Autodesk Inventor part; units mm, degrees
ref_plane "YZ Plane" through (0, 0, 0) normal (1, 0, 0) x (0, 1, 0)
ref_plane "XZ Plane" through (0, 0, 0) normal (0, 1, 0) x (-1, 0, 0)
ref_plane "XY Plane" through (0, 0, 0) normal (0, 0, 1) x (1, 0, 0)
sketch "Sketch1" plane through (0, 0, 0) normal (0, 0, 1) x (1, 0, 0)
  line L0 (0, 0) -> (25, 0)
  line L1 (25, 0) -> (25, 3)
  line L2 (0, 3) -> (25, 3)
  line L3 (0, 0) -> (0, 3)
  line L4 (25, 0) -> (50, 0)
  line L5 (50, 0) -> (50, 3)
  line L6 (25, 3) -> (50, 3)
  line L7 (25, 0) -> (25, 3)
  line L8 (50, 0) -> (75, 0)
  line L9 (75, 0) -> (75, 3)
  line L10 (50, 3) -> (75, 3)
  line L11 (50, 0) -> (50, 3)
  line L12 (0, 0) -> (0, 75)
  line L13 (0, 75) -> (75, 75)
  line L14 (75, 75) -> (75, 0)
  line L15 (75, 0) -> (50, 0)
  line L16 (50, 3) -> (50, 0)
  line L17 (50, 3) -> (25, 3)
  line L18 (25, 3) -> (25, 0)
  line L19 (25, 0) -> (0, 0)
  line L20 (0, 0) -> (0, 25)
  line L21 (0, 25) -> (3, 25)
  line L22 (3, 25) -> (3, 50)
  line L23 (3, 50) -> (0, 50)
  line L24 (25, 75) -> (25, 72)
  line L25 (25, 72) -> (50, 72)
  line L26 (50, 75) -> (50, 72)
  line L27 (75, 50) -> (72, 50)
  line L28 (72, 50) -> (72, 25)
  line L29 (72, 25) -> (75, 25)
  dimension "d0" = 75
  dimension "d1" = 75
  dimension "d2" = 25
  dimension "d3" = 3
  dimension "d4" = 25
  dimension "d5" = 3
  dimension "d6" = 3
extrude "Extrusion1" add sketch "Sketch1" along normal blind 3 contours L3 L2 L1 L0 | L12 L21 L22 L23 L13 L24 L25 L26 L14 L27 L28 L29 L10 L6 L2 | L5 L10 L9 L8
sketch "Sketch2" plane through (0, 0, 0) normal (0, 0, -1) x (-1, 0, 0)
  circle A0 centre (-72, 55.2929) radius 1.5
  circle A1 centre (-20, 68.5) radius 1.5
  circle A2 centre (-23, 21.5) radius 1.5
  circle A3 centre (-72, 23.7071) radius 1.5
  point P0 (0, 0)
extrude "Extrusion2" cut sketch "Sketch2" against normal blind 25.4
sketch "Sketch3" plane through (0, 0, 0) normal (0, 0, -1) x (-1, 0, 0)
  line L0 (-50, 72) -> (-39, 72)
  line L1 (-25, 72) -> (-25, 75)
  line L2 (-25, 75) -> (0, 75)
  line L3 (0, 62.5) -> (0, 50)
  line L4 (0, 50) -> (-3, 50)
  line L5 (-3, 50) -> (-3, 39)
  line L6 (-3, 25) -> (0, 25)
  line L7 (0, 25) -> (0, 0)
  line L8 (0, 0) -> (-25, 0)
  line L9 (-25, 0) -> (-25, 3)
  line L10 (-25, 3) -> (-36, 3)
  line L11 (-50, 3) -> (-50, 0)
  line L12 (-50, 0) -> (-75, 0)
  line L13 (-75, 0) -> (-75, 25)
  line L14 (-75, 25) -> (-72, 25)
  line L15 (-72, 25) -> (-72, 36)
  line L16 (-72, 50) -> (-75, 50)
  line L17 (-75, 62.5) -> (-75, 75)
  line L18 (-75, 75) -> (-50, 75)
  line L19 (-50, 75) -> (-50, 72)
  circle A0 centre (-19, 19.65) radius 1.5
  circle A1 centre (-19, 56.95) radius 1.5
  circle A2 centre (-56.3, 56.95) radius 1.5
  circle A3 centre (-56.3, 19.65) radius 1.5
  line L20 (-39, 72) -> (-36, 72)
  line L21 (-3, 39) -> (-3, 36)
  line L22 (-3, 50) -> (-3, 25)
  line L23 (-39, 3) -> (-36, 3)
  line L24 (-25, 3) -> (-50, 3)
  line L25 (-72, 36) -> (-72, 39)
  line L26 (-72, 25.2071) -> (-72, 50)
  line L27 (-72, 39) -> (-72, 50)
  line L28 (-36, 72) -> (-25, 72)
  line L29 (-3, 36) -> (-3, 25)
  line L30 (-39, 3) -> (-50, 3)
  line L31 (-72, 36) -> (-65.65, 36)
  line L32 (-65.65, 36) -> (-65.65, 34)
  line L33 (-65.65, 34) -> (-63.15, 34)
  line L34 (-63.15, 34) -> (-63.15, 36)
  line L35 (-63.15, 36) -> (-59.3, 36)
  line L36 (-59.3, 36) -> (-59.3, 39)
  line L37 (-59.3, 39) -> (-63.15, 39)
  line L38 (-63.15, 39) -> (-63.15, 41)
  line L39 (-63.15, 41) -> (-65.65, 41)
  line L40 (-65.65, 41) -> (-65.65, 39)
  line L41 (-65.65, 39) -> (-72, 39)
  line L42 (-39, 72) -> (-39, 65.65)
  line L43 (-39, 65.65) -> (-41, 65.65)
  line L44 (-41, 65.65) -> (-41, 63.15)
  line L45 (-41, 63.15) -> (-39, 63.15)
  line L46 (-39, 63.15) -> (-39, 59.3)
  line L47 (-39, 59.3) -> (-36, 59.3)
  line L48 (-36, 59.3) -> (-36, 63.15)
  line L49 (-36, 63.15) -> (-34, 63.15)
  line L50 (-34, 63.15) -> (-34, 65.65)
  line L51 (-34, 65.65) -> (-36, 65.65)
  line L52 (-36, 65.65) -> (-36, 72)
  line L53 (-3, 39) -> (-9.35, 39)
  line L54 (-9.35, 39) -> (-9.35, 41)
  line L55 (-9.35, 41) -> (-11.85, 41)
  line L56 (-11.85, 41) -> (-11.85, 39)
  line L57 (-11.85, 39) -> (-15.7, 39)
  line L58 (-15.7, 39) -> (-15.7, 36)
  line L59 (-15.7, 36) -> (-11.85, 36)
  line L60 (-11.85, 36) -> (-11.85, 34)
  line L61 (-11.85, 34) -> (-9.35, 34)
  line L62 (-9.35, 34) -> (-9.35, 36)
  line L63 (-9.35, 36) -> (-3, 36)
  line L64 (-36, 3) -> (-36, 9.35)
  line L65 (-36, 9.35) -> (-34, 9.35)
  line L66 (-34, 9.35) -> (-34, 11.85)
  line L67 (-34, 11.85) -> (-36, 11.85)
  line L68 (-36, 11.85) -> (-36, 15.7)
  line L69 (-36, 15.7) -> (-39, 15.7)
  line L70 (-39, 15.7) -> (-39, 11.85)
  line L71 (-39, 11.85) -> (-41, 11.85)
  line L72 (-41, 11.85) -> (-41, 9.35)
  line L73 (-41, 9.35) -> (-39, 9.35)
  line L74 (-39, 9.35) -> (-39, 3)
  line L75 (-75, 50) -> (-75, 62.5)
  circle A4 centre (-73.5, 62.5) radius 1.5
  line L76 (0, 75) -> (0, 62.5)
  circle A5 centre (-1.5, 62.5) radius 1.5
extrude "Extrusion3" cut sketch "Sketch3" against normal blind 25.4 contours L20 L52 L51 L50 L49 L48 L47 L46 L45 L44 L43 L42 | L41 L40 L39 L38 L37 L36 L35 L34 L33 L32 L31 L25 | L21 L63 L62 L61 L60 L59 L58 L57 L56 L55 L54 L53 | L74 L73 L72 L71 L70 L69 L68 L67 L66 L65 L64 L23
sketch "Sketch4" plane through (0, 0, 0) normal (0, 0, -1) x (-1, 0, 0)
  line L0 (-75, 61) -> (-75, 64)
  line L1 (0, 65) -> (0, 61.8364)
  line L2 (-75, 62.5) -> (-73.5, 62.5)
  line L3 (0, 63.4182) -> (-1.5, 63.4182)
  circle A0 centre (-73.5, 62.5) radius 1.5
  circle A1 centre (-1.5, 63.4182) radius 1.5
  point P0 (0, 0)
  dimension "d13" = 1.5
  dimension "d14" = 1.5
  dimension "d15" = 3
extrude "Extrusion4" cut sketch "Sketch4" against normal blind 25.4
sketch "Sketch5" plane through (75, 75, 3) normal (1, 0, 0) x (0, 0, -1)
  line L0 (3, -12.5) -> (0, -12.5)
  line L1 (3, -12.5) -> (3, 0)
  line L2 (3, 0) -> (0, 0)
  line L3 (0, -12.5) -> (0, 0)
  line L4 (0, -25) -> (0, -12.5)
  line L5 (3, -25) -> (0, -25)
  line L6 (3, -25) -> (3, -12.5)
  point P0 (3, -75)
extrude "Extrusion5" add sketch "Sketch5" along normal blind 0.5
sketch "Sketch6" plane through (0, 75, 0) normal (-1, 0, 0) x (0, 0, 1)
  line L0 (0, -11.5818) -> (3, -11.5818)
  line L1 (3, 0) -> (3, -11.5818)
  line L2 (0, 0) -> (3, 0)
  line L3 (0, 0) -> (0, -11.5818)
  line L4 (0, -11.5818) -> (0, -25)
  line L5 (0, -25) -> (3, -25)
  line L6 (3, -11.5818) -> (3, -25)
  point P0 (0, -75)
extrude "Extrusion6" add sketch "Sketch6" along normal blind 0.5
properties part number "pared lateral"
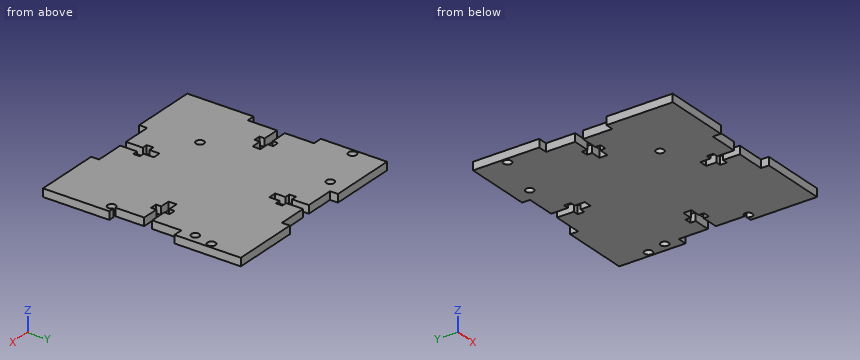
Design review of the part built by this model. Coordinates are the model's own, in mm. Coordinates: 2 decimals unless noted, no trailing zeros. Write each loop counter-clockwise with the first axis right and the second up, starting at its lowest first coordinate (ties: lowest second). Pieces come first, ordered by that corner, then holes.
1) Add section A-A (x = 20). Write out the cut boundary in (y, z).
2) Insertion check: pin 1 (0.9 mm diameter, centred on y = 1.5, z = 2, fed in from +X); pin 2 (1.5 mm diameter, centred on x = 32, z = 1.5, fed in from +Y); pin 3 (0.6 mm diameter, centred on y = 34.5, z = 1, fed in from +X). Each pin has a flat end and moves straight along its axis. Give the tip position at first contact, or say it passes through.
3) Add section B-B (y = 68.5). Write out the cut boundary in (x, z), plus the area to 3 significant figures.
4) To check wall thickness, follow L1, parallel to X at y = 68.5, z = 1.8; L2, parallel to X at y = 10, z = 1.1; L3, parallel to X at y = 60.5, z = 0.65. State the ranges of each line that lie inside material, in increasing order.
5) Add section D-D (z = 1.9). State how many separate pieces and enclosed holes the cut face has, plus the area to 3 significant figures.
6) Add section C-C (x = 43.5). Write out the cut boundary in (y, z), plus the area to 3 significant figures.
Check result:
1. outline: (0, 0) - (67, 0) - (67, 3) - (0, 3) - close; (70, 0) - (75, 0) - (75, 3) - (70, 3) - close
2. pin 1: stops at x = 75
2. pin 2: stops at y = 72
2. pin 3: stops at x = 72
3. outline: (-0.5, 0) - (18.5, 0) - (18.5, 3) - (-0.5, 3) - close; (21.5, 0) - (36, 0) - (36, 3) - (21.5, 3) - close; (39, 0) - (75.5, 0) - (75.5, 3) - (39, 3) - close
3. area: 210 mm2
4. L1: x = -0.5 to 18.5, 21.5 to 36, 39 to 75.5
4. L2: x = 0 to 34, 41 to 75
4. L3: x = -0.5 to 36, 39 to 75.5
5. separate pieces: 1
5. enclosed holes: 5
5. area: 5,120 mm2
6. outline: (3, 0) - (72, 0) - (72, 3) - (3, 3) - close
6. area: 207 mm2
